Could you check a few things on this model? Use its own coordinates, in mm. A direction names the side the tool comes from. Coordinates: 2 decimals unless noted, no trailing zeros. Loops run counter-clockwise (first coordinate to the right, second up) from the corner with the lowest first, then second, coordinate; pieces in that order, holes last. Notation, with made-up numbers: (54, 88.5) - (69, 88.5) arc R5 ccw to (69, 95.5) - close; hole circle Ø4 at (-6.75, -30). An arc over 180 degrees is marked (long way). Put each result on its own line as item: value. Start each with the question number.
```python
from build123d import *

# Parameters (mm, degrees)
SKETCH1_R           = 1
BOSS_EXTRUDE1_DEPTH = 1.6
SKETCH2_R           = 3.25
BOSS_EXTRUDE2_DEPTH = 7.5


with BuildPart() as part:
    # Sketch1 → Boss-Extrude1 (new body)
    with BuildSketch(Plane.XY):
        with BuildLine():
            Line((-10.9, 10.7), (-10.9, -10.7))
            Line((-10.9, -10.7), (-10.9, -12.5))
            ThreePointArc((-10.9, -12.5), (-9.1, -14.3), (-7.3, -12.5))
            Line((-7.3, -12.5), (-7.3, -10.7))
            Line((-7.3, -10.7), (7.3, -10.7))
            Line((7.3, -10.7), (7.3, -12.5))
            ThreePointArc((7.3, -12.5), (9.1, -14.3), (10.9, -12.5))
            Line((10.9, -12.5), (10.9, -10.7))
            Line((10.9, -10.7), (10.9, 10.7))
            Line((10.9, 10.7), (10.9, 12.5))
            ThreePointArc((10.9, 12.5), (9.1, 14.3), (7.3, 12.5))
            Line((7.3, 12.5), (7.3, 10.7))
            Line((7.3, 10.7), (-7.3, 10.7))
            Line((-7.3, 10.7), (-7.3, 12.5))
            ThreePointArc((-7.3, 12.5), (-9.1, 14.3), (-10.9, 12.5))
            Line((-10.9, 12.5), (-10.9, 10.7))
        make_face()
        with Locations((-9.1, 12.5)):
            Circle(SKETCH1_R, mode=Mode.SUBTRACT)
        with Locations(Location((9.1, 12.5, 0), (0, 0, 180))):
            Circle(SKETCH1_R, mode=Mode.SUBTRACT)
        with Locations((9.1, -12.5)):
            Circle(SKETCH1_R, mode=Mode.SUBTRACT)
        with Locations(Location((-9.1, -12.5, 0), (0, 0, 180))):
            Circle(SKETCH1_R, mode=Mode.SUBTRACT)
    extrude(amount=BOSS_EXTRUDE1_DEPTH)

    # Sketch2 → Boss-Extrude2 (add)
    with BuildSketch(Plane.XY.offset(1.6)):
        with Locations(Location((-6.9, -6.2, 0), (0, 0, 180))):
            Circle(SKETCH2_R)
    extrude(amount=BOSS_EXTRUDE2_DEPTH)


solid = part.part
```
(1) I need wall thicknesses on L1, parallel to Y at x = -9.1, z = 1.2; L2, parallel to Z at x = -7.75, y = 7.5; L3, parallel to X at y = -6, z = 7.5. Which ranges of each line are inside material? Lowest first, please. Write a range as [from, to].
(2) I want a section at A-A on x = 9.1. List the corners of the cut face in (y, z) for me, and give its area (3 significant figures).
(3) I want a section at C-C on y = -6.2. List the corners of the cut face in (x, z) for me, and give its area (3 significant figures).
(4) For pin 1 Ø3 at (x, y) = (9.1, -12.5) entering from +Z; pin 2 Ø10 at (x, y) = (-2, 7.5) entering from -Z; pin 3 Ø2 at (x, z) = (-8, 3.5) entering from -Y; pin 4 Ø1.8 at (x, z) = (0, 0.5) entering from -Y, each with a flat end and sliding along its axis, tell me the tip position at first contact or that it passes through.
(5) Which directions (+Z, -Z, +X, -X, +Y, -Y) give clear straight access to the entire face, cutting with the end or side of a thin tool? Please do faces 1 (the flat face through (7.3, -12, 1)), 2 (the flat face through (0, 10.7, 1)), 3 (the flat face through (0, 0, 0)), 4 (the cylindrical face through (-4.321, -4.222, 5.297)).
(6) I want a section at D-D on z = 6.75. List the corners of the cut face in (x, y) for me.
(7) I want a section at B-B on x = -6.9. List the corners of the cut face in (y, z) for me, and give its area (3 significant figures).
Answer sheet:
1. L1: y = [-14.3, -13.5], [-11.5, 11.5], [13.5, 14.3]
1. L2: z = [0, 1.6]
1. L3: x = [-10.14, -3.66]
2. outline: (-14.3, 0) - (-13.5, 0) - (-13.5, 1.6) - (-14.3, 1.6) - close; (-11.5, 0) - (11.5, 0) - (11.5, 1.6) - (-11.5, 1.6) - close; (13.5, 0) - (14.3, 0) - (14.3, 1.6) - (13.5, 1.6) - close
2. area: 39.4 mm^2
3. outline: (-10.9, 0) - (10.9, 0) - (10.9, 1.6) - (-3.65, 1.6) - (-3.65, 9.1) - (-10.15, 9.1) - (-10.15, 1.6) - (-10.9, 1.6) - close
3. area: 83.6 mm^2
4. pin 1: stops at z = 1.6
4. pin 2: stops at z = 0
4. pin 3: stops at y = -9.45
4. pin 4: stops at y = -10.7
5. face 1: +Z, -Z, -Y
5. face 2: +Z, -Z, +Y
5. face 3: -Z, +X, -X, +Y, -Y
5. face 4: +Z
6. outline: circle Ø6.5 at (-6.9, -6.2)
7. outline: (-10.7, 0) - (10.7, 0) - (10.7, 1.6) - (-2.95, 1.6) - (-2.95, 9.1) - (-9.45, 9.1) - (-9.45, 1.6) - (-10.7, 1.6) - close
7. area: 83.0 mm^2
